```python
from build123d import *

# Parameters (mm, degrees)
RESSALTO_EXTRUS_O1_DEPTH = 3
ESBO_O2_R                = 0.8
CORTE_EXTRUS_O1_DEPTH    = 4
CORTE_EXTRUS_O2_DEPTH    = 10


with BuildPart() as part:
    # Esboço1 → Ressalto-extrusão1 (new body)
    with BuildSketch(Plane.XY):
        with BuildLine():
            Line((4.586855285, 67.236842105), (99.586855285, 67.236842105))
            ThreePointArc((99.586855285, 67.236842105), (110.193457003, 62.843443823), (114.586855285, 52.236842105))
            Line((114.586855285, 52.236842105), (114.586855285, 12.236842105))
            ThreePointArc((114.586855285, 12.236842105), (110.193457003, 1.630240387), (99.586855285, -2.763157895))
            Line((99.586855285, -2.763157895), (4.586855285, -2.763157895))
            ThreePointArc((4.586855285, -2.763157895), (-6.019746433, 1.630240387), (-10.413144715, 12.236842105))
            Line((-10.413144715, 12.236842105), (-10.413144715, 52.236842105))
            ThreePointArc((-10.413144715, 52.236842105), (-6.019746433, 62.843443823), (4.586855285, 67.236842105))
        make_face()
    extrude(amount=RESSALTO_EXTRUS_O1_DEPTH)

    # Esboço2 → Corte-extrusão1 (cut, through all)
    with BuildSketch(Plane(origin=(0, 0, 0), x_dir=(-1, 0, 0), z_dir=(0, 0, -1))):
        with Locations((-102.836855285, 53.456842105)):
            Circle(ESBO_O2_R)
    extrude(amount=-CORTE_EXTRUS_O1_DEPTH, mode=Mode.SUBTRACT)

    # Esboço3 → Corte-extrusão2 (cut)
    with BuildSketch(Plane(origin=(0, 0, 0), x_dir=(-1, 0, 0), z_dir=(0, 0, -1))):
        with BuildLine():
            Line((-14.586855285, 7.236842105), (-24.586855285, 7.236842105))
            ThreePointArc((-24.586855285, 7.236842105), (-28.122389191, 8.701308199), (-29.586855285, 12.236842105))
            Line((-29.586855285, 12.236842105), (-29.586855285, 52.236842105))
            ThreePointArc((-29.586855285, 52.236842105), (-28.122389191, 55.772376011), (-24.586855285, 57.236842105))
            Line((-24.586855285, 57.236842105), (-14.586855285, 57.236842105))
            ThreePointArc((-14.586855285, 57.236842105), (-11.051321379, 55.772376011), (-9.586855285, 52.236842105))
            Line((-9.586855285, 52.236842105), (-9.586855285, 12.236842105))
            ThreePointArc((-9.586855285, 12.236842105), (-11.051321379, 8.701308199), (-14.586855285, 7.236842105))
        make_face()
        with BuildLine():
            Line((-47.086855285, 7.236842105), (-57.086855285, 7.236842105))
            ThreePointArc((-57.086855285, 7.236842105), (-60.622389191, 8.701308199), (-62.086855285, 12.236842105))
            Line((-62.086855285, 12.236842105), (-62.086855285, 52.236842105))
            ThreePointArc((-62.086855285, 52.236842105), (-60.622389191, 55.772376011), (-57.086855285, 57.236842105))
            Line((-57.086855285, 57.236842105), (-47.086855285, 57.236842105))
            ThreePointArc((-47.086855285, 57.236842105), (-43.551321379, 55.772376011), (-42.086855285, 52.236842105))
            Line((-42.086855285, 52.236842105), (-42.086855285, 12.236842105))
            ThreePointArc((-42.086855285, 12.236842105), (-43.551321379, 8.701308199), (-47.086855285, 7.236842105))
        make_face()
        with BuildLine():
            Line((-79.586855285, 7.236842105), (-89.586855285, 7.236842105))
            ThreePointArc((-89.586855285, 7.236842105), (-93.122389191, 8.701308199), (-94.586855285, 12.236842105))
            Line((-94.586855285, 12.236842105), (-94.586855285, 52.236842105))
            ThreePointArc((-94.586855285, 52.236842105), (-93.122389191, 55.772376011), (-89.586855285, 57.236842105))
            Line((-89.586855285, 57.236842105), (-79.586855285, 57.236842105))
            ThreePointArc((-79.586855285, 57.236842105), (-76.051321379, 55.772376011), (-74.586855285, 52.236842105))
            Line((-74.586855285, 52.236842105), (-74.586855285, 12.236842105))
            ThreePointArc((-74.586855285, 12.236842105), (-76.051321379, 8.701308199), (-79.586855285, 7.236842105))
        make_face()
    extrude(amount=-CORTE_EXTRUS_O2_DEPTH, mode=Mode.SUBTRACT)


solid = part.part
```
CAD build for the part. Positions are in the model's coordinates, mm. A direction names the side the tool comes from. Coordinates: 2 decimals unless noted, no trailing zeros. Order: outer loops, then holes, each group sorted by start corner. A loop starts at its lowest first (then second) coordinate and runs counter-clockwise, first axis right, second up. Notation, with made-up numbers: M 50,37 L 106,37 A20 cw 106,58 Z; hole C 26,-32 d9. An arc over 180 degrees is marked long. Answer as CSV lines item,"result".
1) Cut at B-B (x = 53.5). List the corners of the cut face in (y, z).
Verdict:
outline,"M -2.76,0 L 7.24,0 L 7.24,3 L -2.76,3 Z; M 57.24,0 L 67.24,0 L 67.24,3 L 57.24,3 Z"
2) Flat gauge pin, fed straight in: P1, Ø1, axis at x = 102.84, y = 53.46, coming from the +Z side. Where does the tip first touch, or does it go through?
Verdict:
P1,"through"
3) Cut at C-C (z = 2). Give the number of separate pieces and of enclosed holes in the cut face, then the cut area to 3 significant figures.
Verdict:
separate pieces,"1"
enclosed holes,"4"
area,"5,620 mm2"
4) Cut at D-D (y = 56). List the corners of the cut face in (x, z), then the cut area to 3 significant figures.
Verdict:
outline,"M -9.93,0 L 11.29,0 L 11.29,3 L -9.93,3 Z; M 27.88,0 L 43.79,0 L 43.79,3 L 27.88,3 Z; M 60.38,0 L 76.29,0 L 76.29,3 L 60.38,3 Z; M 92.88,0 L 114.11,0 L 114.11,3 L 92.88,3 Z"
area,"223 mm2"
5) Mould opens along X. For faces 3 (the flat face through (114.587, 33, 1)), 4 (the cylindrical face through (43.59, 55.81, 1.48)), 5 (the cylindrical face through (-5.9, 1.51, 1.48)) say: released by +X, released by -X, zero draft, split by the parting line, or undercut.
Verdict:
face 3,"released by +X"
face 4,"undercut"
face 5,"released by -X"
6) Cut at A-A (y = 18). List the corners of the cut face in (x, z), then the cut area to 3 significant figures.
Verdict:
outline,"M -10.41,0 L 9.59,0 L 9.59,3 L -10.41,3 Z; M 29.59,0 L 42.09,0 L 42.09,3 L 29.59,3 Z; M 62.09,0 L 74.59,0 L 74.59,3 L 62.09,3 Z; M 94.59,0 L 114.59,0 L 114.59,3 L 94.59,3 Z"
area,"195 mm2"
7) Drill centre lines: L1, parallel to X at y = 28.5, z = 1.45; L2, parallel to X at y = 53, z = 1.5; L3, parallel to Y at x = 88.5, z = 0.6. Where is each one in solid material? Low to high. Write a range as from..to.
Verdict:
L1,"-10.41..9.59, 29.59..42.09, 62.09..74.59, 94.59..114.59"
L2,"-10.39..9.65, 29.53..42.15, 62.03..74.65, 94.53..102.18, 103.49..114.57"
L3,"-2.76..7.24, 57.24..67.24"
8) 3-axis set-ups, long thin cutter, end or side, ignore diameter. For faces 1 (the flat face through (62.087, 32, 1)), 2 (the flat face through (51, 67.237, 1)): which of +Z, -Z, +X, -X, +Y, -Y reach the whole face in a straight line?
Verdict:
face 1,"+Z, -Z"
face 2,"+Z, -Z, +X, -X, +Y"
